Autodesk Inventor part; units mm, degrees
ref_plane "YZ Plane" through (0, 0, 0) normal (1, 0, 0) x (0, 1, 0)
ref_plane "XZ Plane" through (0, 0, 0) normal (0, 1, 0) x (-1, 0, 0)
ref_plane "XY Plane" through (0, 0, 0) normal (0, 0, 1) x (1, 0, 0)
sketch "Skizze1" plane through (0, 0, 0) normal (0, 0, 1) x (1, 0, 0)
  line L0 (-6.35, 3.429) -> (6.35, 3.429)
  line L1 (6.35, 3.429) -> (6.35, -3.429)
  line L2 (6.35, -3.429) -> (-6.35, -3.429)
  line L3 (-6.35, -3.429) -> (-6.35, 3.429)
  point P0 (0, 0)
  point P1 (6.35, 0)
  point P2 (0, -3.429)
  dimension "d0" = 12.7
  dimension "d1" = 6.858
extrude "Extrusion1" add sketch "Skizze1" along normal blind 8.89
sketch "Skizze2" plane through (0, 0, 8.89) normal (0, 0, 1) x (1, 0, 0)
  circle A0 centre (0, 0) radius 2.5
  circle A1 centre (0, 0) radius 2.25
  dimension "d4" = 5
  dimension "d10" = 4.5
extrude "Extrusion2" add sketch "Skizze2" along normal blind 8.89 contours A0 | A1
thread "Gewinde1"
fillet "Rundung1" radius 0.25 1 edges at (-2.5, 0, 17.78)
sketch "Skizze3" plane through (0, 0, 17.78) normal (0, 0, 1) x (1, 0, 0)
  circle A0 centre (0, 0) radius 2.25
  circle A1 centre (0, 0) radius 2
  dimension "d11" = 4
extrude "Extrusion3" cut sketch "Skizze3" against normal blind 5 contours A1
sketch "Skizze4" plane through (0, 0, 12.78) normal (0, 0, 1) x (1, 0, 0)
  circle A0 centre (0, 0) radius 2
  circle A1 centre (0, 0) radius 1.46
  dimension "d14" = 2.92
extrude "Extrusion4" add sketch "Skizze4" along normal blind 10.67 contours A1
fillet "Rundung3" radius 0.25 12 edges at (0, 3.429, 8.89) (-6.35, 0, 8.89) (0, -3.429, 8.89) (6.35, 0, 8.89) (-6.35, 0, 0) (-6.35, -3.429, 4.445) (-6.35, 3.429, 4.445) (6.35, 3.429, 4.445) (0, 3.429, 0) (6.35, -3.429, 4.445) (0, -3.429, 0) (6.35, 0, 0)
fillet "Rundung5" radius 1 1 edges at (-1.46, 0, 23.45)
properties part number "Schalter"
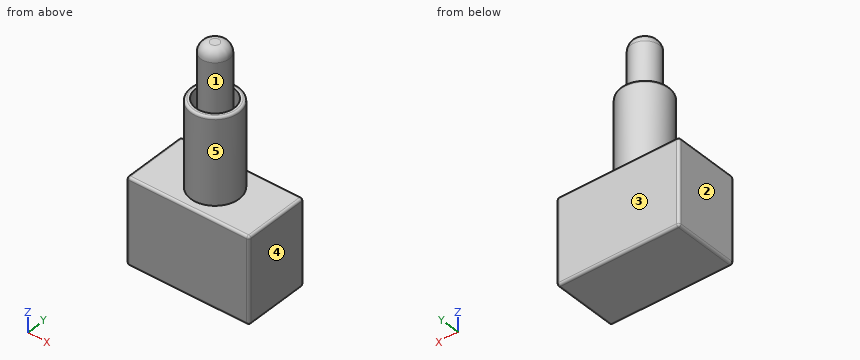
The listing builds one solid part. Answer for the finished solid, in the listing's coordinates (mm). Face numbers are marked on the shaded views. A direction names the side the tool comes from. Give positions to 0.01 mm unless a question says otherwise; leave off trailing zeros. Loops run counter-clockwise (first coordinate to the right, second up) from the corner with the lowest first, then second, coordinate; pieces in that order, holes last. Notation, with made-up numbers: (-37.5, -26.5) - (-14.5, -26.5) arc R20 ccw to (-14.5, -6.5) - close; hole circle Ø1 at (27.5, 84.5). An arc over 180 degrees is marked (long way). Answer as CSV lines item,"result". Start each with the question number.
Item 1: Find the intervals of material crossed by line 1 (Y direction, x = 0, z = 14); line 2 (Y direction, x = -0.75, z = 14.75); line 3 (Z direction, x = 4.25, y = -2), in increasing order. Write a range as from..to.
Item 2: Each of these flat-tipped pins is pushed along its axis until it touches: pin 1 (1 mm diameter, centred on x = 0.5, z = 19, fed in from -Y); pin 2 (1.9 mm diameter, centred on x = -0.5, y = -1.5, fed in from +Z); pin 3 (4 mm diameter, centred on x = 1, z = 13.5, fed in from +Y). Where does it stop, or does it pass through?
Item 3: For the marked faces 4 and 5, determine the directions among +Z, -Z, +X, -X, +Y, -Y from which every point of the face is accessible in a straight line to the end or side of a thin tool.
Item 4: A cutting plane is placed at A-A on x = -3.5. Determine the outline of the cut face in (y, z), then the cut area to 3 significant figures.
Item 5: A cutting plane is placed at C-C on z = 20.25. Determine the outline of the cut face in (x, y).
Item 6: A cutting plane is placed at B-B on z = 12.25. Determine the outline of the cut face in (x, y), then the cut area to 3 significant figures.
Item 7: The mould has two halves that part along Y. Classify the marked faces 1, 2 and 3: +Y half, -Y half, draft (parallel to the pull), parting line (faces both ways), or undercut.
Found:
1,line 1,"y = -2.5..-2, -1.46..1.46, 2..2.5"
1,line 2,"y = -2.38..-1.85, -1.25..1.25, 1.85..2.38"
1,line 3,"z = 0..8.89"
2,pin 1,"stops at y = -1.46"
2,pin 2,"stops at z = 23.44"
2,pin 3,"stops at y = 2.5"
3,face 4,"+Z, -Z, +X, +Y, -Y"
3,face 5,"+Z"
4,outline,"(-3.43, 0.25) arc R0.25 ccw to (-3.18, 0) - (3.18, 0) arc R0.25 ccw to (3.43, 0.25) - (3.43, 8.64) arc R0.25 ccw to (3.18, 8.89) - (-3.18, 8.89) arc R0.25 ccw to (-3.43, 8.64) - close"
4,area,"60.9 mm^2"
5,outline,"circle Ø2.92 at (0, 0)"
6,outline,"circle Ø5 at (0, 0)"
6,area,"19.6 mm^2"
7,face 1,"undercut"
7,face 2,"draft"
7,face 3,"+Y half"
